Here's the drawing with two shaded views (mm, measured from the low corner). I have some questions. A direction names the side the tool comes from. Coordinates: 2 decimals unless noted, no trailing zeros. Order: outer loops, then holes, each group sorted by start corner. A loop starts at its lowest first (then second) coordinate and runs counter-clockwise, first axis right, second up. Notation, with made-up numbers: (6, 62.5) -> (13, 62.5) arc R14 ccw to (13, 77.5) -> close; hole circle Ø1 at (-20.5, 58). An arc over 180 degrees is marked (long way). Write item = value, one per line.
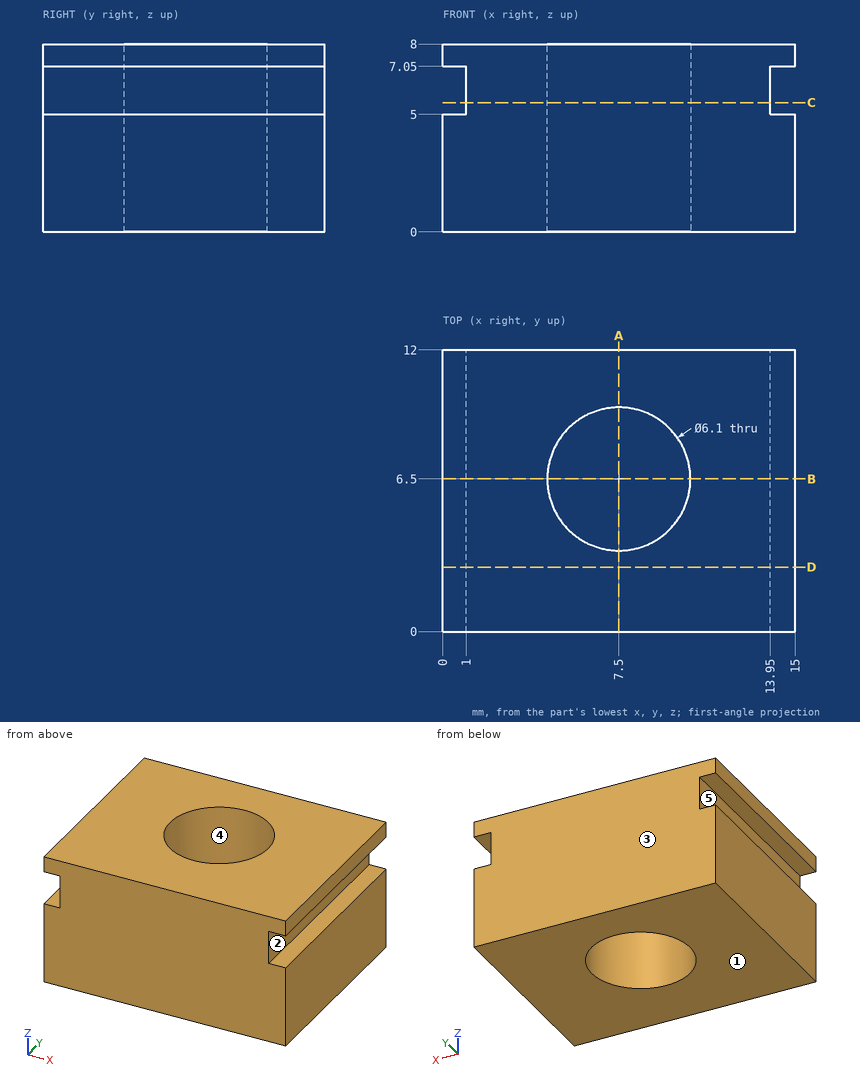
Item 1: I'm going to push flat-ended pins straight in: P1, Ø0.6, axis at y = 3, z = 6, coming from the -X side; P2, Ø1, axis at x = 9.5, y = 8, coming from the -Z side; P3, Ø1, axis at y = 8.5, z = 6.5, coming from the +X side. Where does each tip first touch, or does it pass through?
A:
P1 = 1
P2 = through
P3 = 13.95
Item 2: I want a section at A-A, the plane x = 7.5. Please give me the cut outline in (y, z).
A:
outline = (0, 0) -> (3.45, 0) -> (3.45, 8) -> (0, 8) -> close; (9.55, 0) -> (12, 0) -> (12, 8) -> (9.55, 8) -> close
Item 3: I want a section at C-C, the plane z = 5.5. Please give me the cut outline in (x, y).
A:
outline = (1, 0) -> (13.95, 0) -> (13.95, 12) -> (1, 12) -> close; hole circle Ø6.1 at (7.5, 6.5)
Item 4: If I drill on probe 1 along Y at (x, z) = (7.5, 4.25); probe 2 along Z at (x, y) = (14.25, 10.75); probe 3 along X at (y, z) = (2.25, 6), over which ranges is the centre line in solid material (lowest first)?
A:
probe_1 = 0 to 3.45, 9.55 to 12
probe_2 = 0 to 5, 7.05 to 8
probe_3 = 1 to 13.95
Item 5: If we mould it in two halves opening along Y, with no side actions, what happens to the marked faces 3, 4 and 5? For each: pulls with the +Y half, pulls with the -Y half, needs draft (parallel to the pull), parting line crosses it, or undercut.
A:
face_3 = pulls with the +Y half
face_4 = undercut
face_5 = needs draft
Item 6: For the marked faces 1 and 2, which set-ups out of +Z, -Z, +X, -X, +Y, -Y let a thin tool reach every point of the face, with its end or its side?
A:
face_1 = -Z, +X, -X, +Y, -Y
face_2 = +X, +Y, -Y
Item 7: I want a section at D-D, the plane y = 2.75. Please give me the cut outline in (x, z).
A:
outline = (0, 0) -> (15, 0) -> (15, 5) -> (13.95, 5) -> (13.95, 7.05) -> (15, 7.05) -> (15, 8) -> (0, 8) -> (0, 7.05) -> (1, 7.05) -> (1, 5) -> (0, 5) -> close
Item 8: I want a section at B-B, the plane y = 6.5. Please give me the cut outline in (x, z), plus the area to 3 significant figures.
A:
outline = (0, 0) -> (4.45, 0) -> (4.45, 8) -> (0, 8) -> (0, 7.05) -> (1, 7.05) -> (1, 5) -> (0, 5) -> close; (10.55, 0) -> (15, 0) -> (15, 5) -> (13.95, 5) -> (13.95, 7.05) -> (15, 7.05) -> (15, 8) -> (10.55, 8) -> close
area = 67.0 mm2
